The figure shows three views and two pictorial views of one solid part (mm, origin at its lowest corner). Answer the questions. A direction names the side the tool comes from. Coordinates: 2 decimals unless noted, no trailing zeros. Write each loop counter-clockwise with the first axis right and the second up, starting at its lowest first coordinate (ties: lowest second). Pieces come first, ordered by that corner, then holes. Notation, with made-up numbers: M -7.75,74 L 16.25,74 A20 ccw 16.25,103 Z; hole C -34,70 d7. An arc over 180 degrees is marked long. Answer as CSV lines item,"result".
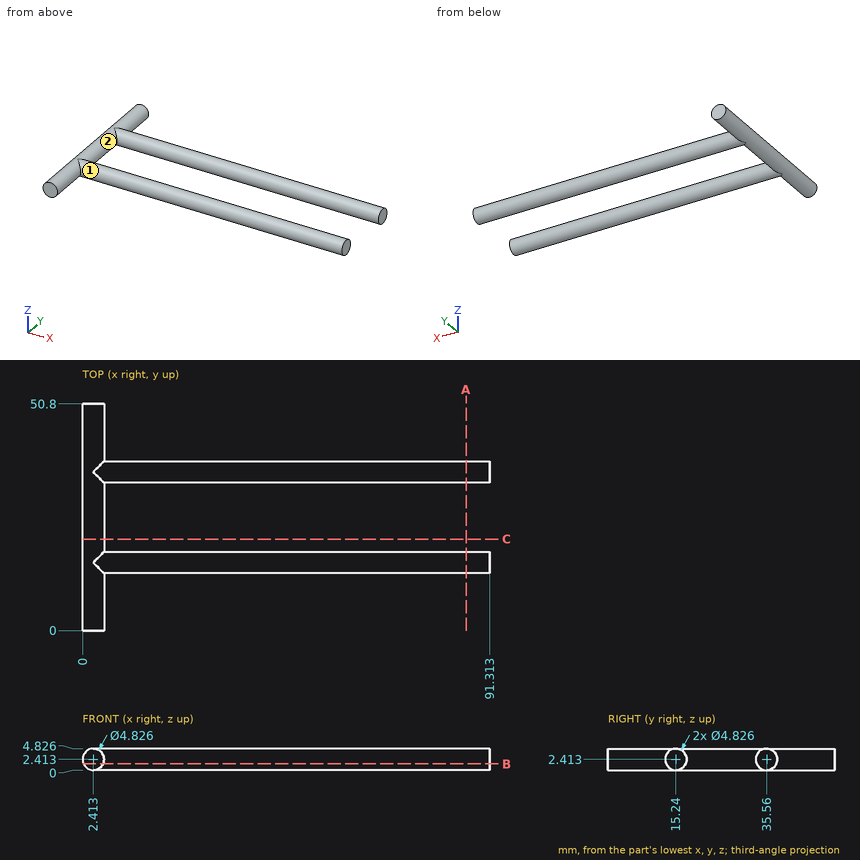
Q1. For the marked faces 1 and 2, determine the directions among +Z, -Z, +X, -X, +Y, -Y from which every point of the face is accessible in a straight line to the end or side of a thin tool.
Output:
face 1,"+X"
face 2,"none"
Q2. Find section C-C (y = 20.5). Give the vertices of the cut face in (x, z), and give its area (3 significant figures).
Output:
outline,"C 2.41,2.41 d4.83"
area,"18.3 mm2"
Q3. Find section A-A (x = 86). Give the vertices of the cut face in (y, z), and give its area (3 significant figures).
Output:
outline,"C 15.24,2.41 d4.83; C 35.56,2.41 d4.83"
area,"36.6 mm2"
Q4. Flat-ended cylindrical pins translate along their axes: pin 1 Ø2 at (x, z) = (70.5, 4) entering from -Y; pin 2 Ø10 at (x, y) = (81.5, 17.5) entering from +Z; pin 3 Ø2 at (y, z) = (29.5, 4) entering from +X. Find the tip coordinate at first contact, or state that the pin passes through.
Output:
pin 1,"y = 12.9"
pin 2,"z = 4.83"
pin 3,"x = 4.75"
Q5. Find section B-B (z = 1.4). Give the vertices of the cut face in (x, y), and give its area (3 significant figures).
Output:
outline,"M 0.22,0 L 4.6,0 L 4.6,13.05 L 91.31,13.05 L 91.31,17.43 L 4.6,17.43 L 4.6,33.37 L 91.31,33.37 L 91.31,37.75 L 4.6,37.75 L 4.6,50.8 L 0.22,50.8 Z"
area,"982 mm2"
Q6. Straight lines are drawn through the part: line 1 (Y direction, x = 15, z = 2.7); line 2 (Y direction, x = 74.5, z = 3.95); line 3 (X direction, y = 39.5, z = 3.35). For each, find the intervals that lie inside material, in ascending order.
Output:
line 1,"12.84 to 17.64, 33.16 to 37.96"
line 2,"13.38 to 17.1, 33.7 to 37.42"
line 3,"0.19 to 4.64"
